For this review, take the finished solid that the model builds, in its own axes (mm). Round coordinates to 2 decimals unless told otherwise and drop trailing zeros. Order: outer loops, then holes, each group sorted by start corner. A loop starts at its lowest first (then second) coordinate and runs counter-clockwise, first axis right, second up. Notation, with made-up numbers: (14.5, 86.5) - (41.5, 86.5) arc R27 cw to (41.5, 111.5) - close; hole circle Ø10 at (53.25, 54.5). An arc over 180 degrees is marked (long way). One line per item, written item: value.
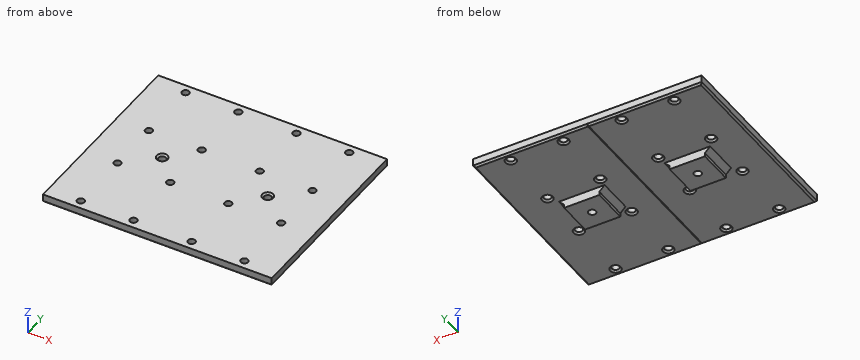
```python
from build123d import *

# Parameters (mm, degrees)
SKETCH_1_W          = 130
SKETCH_1_H          = 110
EXTRUDE_1_DEPTH     = 5
SKETCH_4_R          = 2.05
CUT_EXTRUDE_1_DEPTH = 5
CHAMFER_2_SIZE      = 1
SKETCH_6_W          = 20
SKETCH_6_H          = 20
EXTRUDE_2_DEPTH     = 5
CHAMFER_3_SIZE      = 3
SKETCH_7_R          = 2.1
CUT_EXTRUDE_2_DEPTH = 49
CHAMFER_4_SIZE      = 1
SKETCH_8_W          = 0.5
SKETCH_8_H          = 110
CUT_EXTRUDE_3_DEPTH = 0.5


with BuildPart() as part:
    # 草图1 → 凸台-拉伸1 (new body)
    with BuildSketch(Plane.XY):
        with Locations((65, -55)):
            Rectangle(SKETCH_1_W, SKETCH_1_H)
    extrude(amount=EXTRUDE_1_DEPTH)

    # 草图4 → 切除-拉伸1 (cut)
    with BuildSketch(Plane(origin=(0, 0, 0), x_dir=(-1, 0, 0), z_dir=(0, 0, -1))):
        with Locations((-111.5, -5)):
            Circle(SKETCH_4_R)
        with Locations((-81.5, -5)):
            Circle(SKETCH_4_R)
        with Locations((-111.5, -40)):
            Circle(SKETCH_4_R)
        with Locations((-81.5, -40)):
            Circle(SKETCH_4_R)
        with Locations(Location((-48.5, -40, 0), (0, 0, 180))):
            Circle(SKETCH_4_R)
        with Locations(Location((-18.5, -40, 0), (0, 0, 180))):
            Circle(SKETCH_4_R)
        with Locations(Location((-18.5, -5, 0), (0, 0, 180))):
            Circle(SKETCH_4_R)
        with Locations(Location((-48.5, -5, 0), (0, 0, 180))):
            Circle(SKETCH_4_R)
        with Locations((-48.5, -105)):
            Circle(SKETCH_4_R)
        with Locations((-18.5, -105)):
            Circle(SKETCH_4_R)
        with Locations((-18.5, -70)):
            Circle(SKETCH_4_R)
        with Locations((-48.5, -70)):
            Circle(SKETCH_4_R)
        with Locations(Location((-81.5, -70, 0), (0, 0, 180))):
            Circle(SKETCH_4_R)
        with Locations(Location((-111.5, -70, 0), (0, 0, 180))):
            Circle(SKETCH_4_R)
        with Locations(Location((-81.5, -105, 0), (0, 0, 180))):
            Circle(SKETCH_4_R)
        with Locations(Location((-111.5, -105, 0), (0, 0, 180))):
            Circle(SKETCH_4_R)
    extrude(amount=-CUT_EXTRUDE_1_DEPTH, mode=Mode.SUBTRACT)

    # 倒角2
    chamfer_2_edges = [part.edges().sort_by_distance(p)[0] for p in [
        (50.55, -105, 0),
        (46.45, -5, 0),
        (16.45, -5, 0),
        (16.45, -40, 0),
        (83.55, -5, 0),
        (113.55, -40, 0),
        (83.55, -40, 0),
        (65, 0, 0),
        (46.45, -40, 0),
        (109.45, -70, 0),
        (130, -55, 0),
        (79.45, -105, 0),
        (109.45, -105, 0),
        (65, -110, 0),
        (79.45, -70, 0),
        (50.55, -70, 0),
        (0, -55, 0),
        (20.55, -70, 0),
        (20.55, -105, 0),
        (113.55, -5, 0),
    ]]
    chamfer(chamfer_2_edges, length=CHAMFER_2_SIZE)

    # 草图6 → 凸台-拉伸2 (add)
    with BuildSketch(Plane(origin=(0, 0, 0), x_dir=(-1, 0, 0), z_dir=(0, 0, -1))):
        with Locations((-95, -55)):
            Rectangle(SKETCH_6_W, SKETCH_6_H)
        with Locations((-35, -55)):
            Rectangle(SKETCH_6_W, SKETCH_6_H)
    extrude(amount=EXTRUDE_2_DEPTH)

    # 倒角3
    chamfer_3_edges = [part.edges().sort_by_distance(p)[0] for p in [
        (105, -55, 0),
        (85, -55, 0),
        (45, -55, 0),
        (25, -55, 0),
    ]]
    chamfer(chamfer_3_edges, length=CHAMFER_3_SIZE)

    # 草图7 → 切除-拉伸2 (cut)
    with BuildSketch(Plane(origin=(0, 0, -5), x_dir=(-1, 0, 0), z_dir=(0, 0, -1))):
        with Locations((-95, -55)):
            Circle(SKETCH_7_R)
        with Locations((-35, -55)):
            Circle(SKETCH_7_R)
    extrude(amount=-CUT_EXTRUDE_2_DEPTH, mode=Mode.SUBTRACT)

    # 倒角4
    chamfer_4_edges = [part.edges().sort_by_distance(p)[0] for p in [
        (97.1, -55, 5),
        (37.1, -55, 5),
    ]]
    chamfer(chamfer_4_edges, length=CHAMFER_4_SIZE)

    # 草图8 → 切除-拉伸3 (cut)
    with BuildSketch(Plane(origin=(0, 0, 0), x_dir=(-1, 0, 0), z_dir=(0, 0, -1))):
        with Locations((-65, -55)):
            Rectangle(SKETCH_8_W, SKETCH_8_H)
    extrude(amount=-CUT_EXTRUDE_3_DEPTH, mode=Mode.SUBTRACT)


solid = part.part
```
Item 1: Take a section at D-D (x = 59.5). Write out the cut boundary in (y, z).
Returned:
outline: (-110, 1) - (-109, 0) - (-1, 0) - (0, 1) - (0, 5) - (-110, 5) - close
Item 2: For P1, Ø3.5, axis at x = 81.5, y = -5, coming from the -Z side; P2, Ø5.5, axis at x = 35.5, z = -3, coming from the -Y side; P3, Ø1, axis at y = -55, z = -4, coming from the -X side; P4, Ø6.5, axis at x = 81.5, y = -105, coming from the -Z side, all flat-tipped, find the tip position at first contact; note any pin that passes through.
Returned:
P1: through
P2: y = -65
P3: x = 25
P4: z = 0
Item 3: Take a section at A-A (x = 18.5). Count the separate pieces of the cut face and the enclosed holes in it, plus the area to 3 significant figures.
Returned:
separate pieces: 5
enclosed holes: 0
area: 463 mm^2
Item 4: Wall thickness on line 1 (Y direction, x = 111.5, z = 2); line 2 (Z direction, x = 27, y = -8.5); line 3 (Y direction, x = 35, z = 0.25): over which ranges is each line inside the solid? List them lowest first.
Returned:
line 1: -110 to -107.05, -102.95 to -72.05, -67.95 to -42.05, -37.95 to -7.05, -2.95 to 0
line 2: 0 to 5
line 3: -109.25 to -57.1, -52.9 to -0.75
Item 5: Take a section at C-C (x = 35). Write out the cut boundary in (y, z).
Returned:
outline: (-110, 1) - (-109, 0) - (-65, 0) - (-65, -5) - (-57.1, -5) - (-57.1, 4) - (-58.1, 5) - (-110, 5) - close; (-52.9, -5) - (-45, -5) - (-45, 0) - (-1, 0) - (0, 1) - (0, 5) - (-51.9, 5) - (-52.9, 4) - close
